Work out the finished part from the listing and answer in its coordinate system (mm). Face numbers are marked on the shaded views. A direction names the side the tool comes from. Round coordinates to 2 decimals unless told otherwise and drop trailing zeros. Order: outer loops, then holes, each group sorted by start corner. A loop starts at its lowest first (then second) coordinate and runs counter-clockwise, first axis right, second up. Notation, with made-up numbers: (34, -20.75) -> (74, -20.75) arc R19 cw to (74, -16.75) -> close; hole circle Ø3 at (24, 84). An arc over 180 degrees is marked (long way). Use one line per item in the form item = value.
```python
from build123d import *

# Parameters (mm, degrees)
SKETCH1_R           = 4.5
SKETCH1_R_2         = 2
SKETCH1_R_3         = 2.003539683
SKETCH1_W           = 8
SKETCH1_H           = 5
BOSS_EXTRUDE1_DEPTH = 2.5


with BuildPart() as part:
    # Sketch1 → Boss-Extrude1 (new, symmetric)
    with BuildSketch(Plane.XY):
        with BuildLine():
            Line((-27.5, 0), (27.5, 0))
            ThreePointArc((27.5, 0), (36.5, 9), (27.5, 18))
            Line((27.5, 18), (11.1, 18))
            ThreePointArc((11.1, 18), (4.028932188, 20.928932188), (1.1, 28))
            Line((1.1, 28), (1.1, 33))
            ThreePointArc((1.1, 33), (-6.9, 41), (-14.9, 33))
            Line((-14.9, 33), (-14.9, 22))
            ThreePointArc((-14.9, 22), (-17.828932188, 14.928932188), (-24.9, 12))
            Line((-24.9, 12), (-27.5, 12))
            ThreePointArc((-27.5, 12), (-33.5, 6), (-27.5, 0))
        make_face()
        with Locations((27.5, 9)):
            Circle(SKETCH1_R, mode=Mode.SUBTRACT)
        with Locations((-27.5, 6)):
            Circle(SKETCH1_R_2, mode=Mode.SUBTRACT)
        with Locations((-6.9, 33)):
            Circle(SKETCH1_R_3, mode=Mode.SUBTRACT)
        with Locations((-11.5, 6)):
            Rectangle(SKETCH1_W, SKETCH1_H, mode=Mode.SUBTRACT)
        with Locations((6.5, 6)):
            Rectangle(SKETCH1_W, SKETCH1_H, mode=Mode.SUBTRACT)
    extrude(amount=BOSS_EXTRUDE1_DEPTH, both=True)


solid = part.part
```
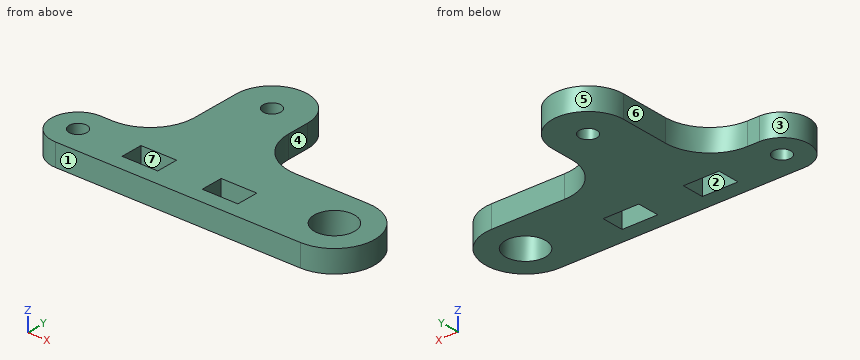
Item 1: The part is cut by section C-C, the plane y = 11. Give the vertices of the cut face in (x, z).
Findings:
outline = (-30.82, -2.5) -> (23.47, -2.5) -> (23.47, 2.5) -> (-30.82, 2.5) -> close; (31.53, -2.5) -> (36.27, -2.5) -> (36.27, 2.5) -> (31.53, 2.5) -> close
Item 2: Consider line 1 along Y through (x, z) = (27.5, 0.6); line 2 along Y through (x, z) = (-8.5, -1.9); line 3 along Y through (x, z) = (-6.9, 1.35). Determine where each line is inside the solid, lowest interval first.
Findings:
line_1 = 0 to 4.5, 13.5 to 18
line_2 = 0 to 3.5, 8.5 to 31.79, 34.21 to 40.84
line_3 = 0 to 31, 35 to 41
Item 3: For the marked faces 4, 5, 6 and 7, determine the directions among +Z, -Z, +X, -X, +Y, -Y from which every point of the face is accessible in a straight line to the end or side of a thin tool.
Findings:
face_4 = +Z, -Z, +X, +Y
face_5 = +Z, -Z, +Y
face_6 = +Z, -Z, -X, +Y
face_7 = +Z, -Z
Item 4: The part is cut by section A-A, the plane x = 29. Give the vertices of the cut face in (y, z), and give its area (3 significant figures).
Findings:
outline = (0.13, -2.5) -> (4.76, -2.5) -> (4.76, 2.5) -> (0.13, 2.5) -> close; (13.24, -2.5) -> (17.87, -2.5) -> (17.87, 2.5) -> (13.24, 2.5) -> close
area = 46.3 mm^2
Item 5: The part is cut by section B-B, the plane z = -1.15. Give the vertices of the cut face in (x, y).
Findings:
outline = (-27.5, 0) -> (27.5, 0) arc R9 ccw to (27.5, 18) -> (11.1, 18) arc R10 cw to (1.1, 28) -> (1.1, 33) arc R8 ccw to (-14.9, 33) -> (-14.9, 22) arc R10 cw to (-24.9, 12) -> (-27.5, 12) arc R6 ccw to start; hole circle Ø4 at (-27.5, 6); hole (-15.5, 3.5) -> (-7.5, 3.5) -> (-7.5, 8.5) -> (-15.5, 8.5) -> close; hole circle Ø4.01 at (-6.9, 33); hole (2.5, 3.5) -> (10.5, 3.5) -> (10.5, 8.5) -> (2.5, 8.5) -> close; hole circle Ø9 at (27.5, 9)
Item 6: Determine the mould class of the marked faces 1, 2 and 3 for opening direction Y: released by +Y, released by -Y, zero draft, split by the parting line, or undercut.
Findings:
face_1 = released by -Y
face_2 = undercut
face_3 = split by the parting line
Item 7: Flat-ended cylindrical pins translate along their axes: P1, Ø2.5, axis at x = -27.5, y = 6, coming from the -Z side; P2, Ø0.8, axis at x = -26, z = 1, coming from the +Y side; P3, Ø3, axis at x = -19, z = -0.5, coming from the -Y side; P4, Ø2.5, axis at x = -12.5, z = 0.5, coming from the +Y side. Find the tip coordinate at first contact, or state that the pin passes through.
Findings:
P1 = through
P2 = 12
P3 = 0
P4 = 39.71
Item 8: The part is cut by section D-D, the plane y = 6. Give the vertices of the cut face in (x, z).
Findings:
outline = (-33.5, -2.5) -> (-29.5, -2.5) -> (-29.5, 2.5) -> (-33.5, 2.5) -> close; (-25.5, -2.5) -> (-15.5, -2.5) -> (-15.5, 2.5) -> (-25.5, 2.5) -> close; (-7.5, -2.5) -> (2.5, -2.5) -> (2.5, 2.5) -> (-7.5, 2.5) -> close; (10.5, -2.5) -> (24.15, -2.5) -> (24.15, 2.5) -> (10.5, 2.5) -> close; (30.85, -2.5) -> (35.99, -2.5) -> (35.99, 2.5) -> (30.85, 2.5) -> close
